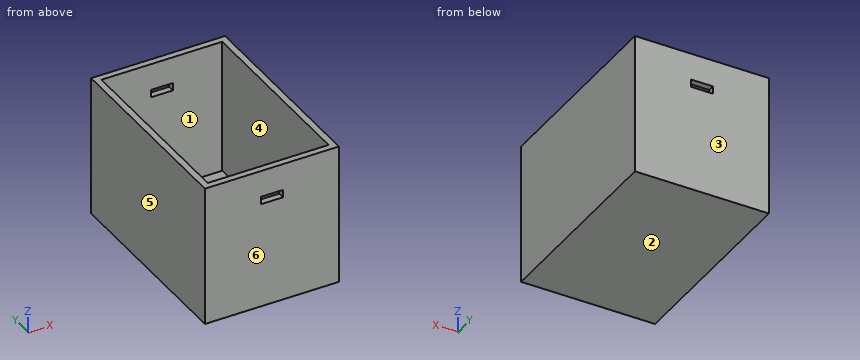
```python
from build123d import *

# Parameters (mm, degrees)
F0_W     = 22
F0_H     = 34
F1_DEPTH = 1.2
F0_W_2   = 24.4
F0_H_2   = 36.4
F2_DEPTH = 25.7
F3_W     = 4
F3_H     = 1.4
F4_DEPTH = 36.401


with BuildPart() as f1:
    # F0 (on Top) → F1 (new body)
    with BuildSketch(Plane.XY):
        Rectangle(F0_W, F0_H)
    extrude(amount=F1_DEPTH)

    # F0 (on Top) → F2 (join)
    with BuildSketch(Plane.XY):
        Rectangle(F0_W_2, F0_H_2)
        Rectangle(F0_W, F0_H, mode=Mode.SUBTRACT)
    extrude(amount=F2_DEPTH)

    # F3 (on face) → F4 (cut, through all)
    with BuildSketch(Plane(origin=(0, 18.2, 0), x_dir=(-1, 0, 0), z_dir=(0, 1, 0))):
        with Locations((0, 20.1)):
            Rectangle(F3_W, F3_H)
    extrude(amount=-F4_DEPTH, mode=Mode.SUBTRACT)


solid = f1.part
```
Part model, mm, in its own coordinate system. Face numbers are marked on the shaded views. A direction names the side the tool comes from. Round coordinates to 2 decimals unless told otherwise and drop trailing zeros. Write each loop counter-clockwise with the first axis right and the second up, starting at its lowest first coordinate (ties: lowest second). Pieces come first, ordered by that corner, then holes. Notation, with made-up numbers: (-6.5, 41) -> (48.5, 41) arc R22 ccw to (48.5, 54) -> close; hole circle Ø5 at (87.5, -4.75). An arc over 180 degrees is marked (long way). Return JSON: item names as keys, results as strings. Group by question number.
Q1. Saw through at D-D on x = 1. Write the cut outline in (y, z).
Q2. Which spindle directions (+Z, -Z, +X, -X, +Y, -Y) get a long thin tool onto all of the face, cutting with end or side? Do the marked faces 1 and 2. Say none if no direction does.
Q3. Mould opens along Y. For the marked faces 3, 4, 5 and 6 say: pulls with the +Y half, pulls with the -Y half, needs draft (parallel to the pull), parting line crosses it, or undercut.
Q4. Saw through at B-B on y = -6. Write the cut outline in (x, z).
Q5. Probe L1, parallel to Y at x = 2.5, z = 18.25; L2, parallel to X at y = -2.5, z = 20.5; L3, parallel to Z at x = -9.75, y = 13. List the from-to ranges inside material, lowest first. Write a range as [from, to].
Q6. Pin check, flat tip, straight feed: pin 1 (2 mm diameter, centred on x = 2, y = 7, fed in from +Z). Stop position of the tip, or through.
Q7. Saw through at A-A on x = 5.25. Write the cut outline in (y, z), plus the area to 3 significant figures.
Q8. Saw through at C-C on z = 6. Write the cut outline in (x, y).
Answer:
{
 "1": {"outline": "(-18.2, 0) -> (18.2, 0) -> (18.2, 19.4) -> (17, 19.4) -> (17, 1.2) -> (-17, 1.2) -> (-17, 19.4) -> (-18.2, 19.4) -> close; (-18.2, 20.8) -> (-17, 20.8) -> (-17, 25.7) -> (-18.2, 25.7) -> close; (17, 20.8) -> (18.2, 20.8) -> (18.2, 25.7) -> (17, 25.7) -> close"},
 "2": {"face 1": "+Z", "face 2": "-Z, +X, -X, +Y, -Y"},
 "3": {"face 3": "pulls with the +Y half", "face 4": "undercut", "face 5": "needs draft", "face 6": "pulls with the -Y half"},
 "4": {"outline": "(-12.2, 0) -> (12.2, 0) -> (12.2, 25.7) -> (11, 25.7) -> (11, 1.2) -> (-11, 1.2) -> (-11, 25.7) -> (-12.2, 25.7) -> close"},
 "5": {"L1": "[-18.2, -17], [17, 18.2]", "L2": "[-12.2, -11], [11, 12.2]", "L3": "[0, 1.2]"},
 "6": {"pin 1": "z = 1.2"},
 "7": {"outline": "(-18.2, 0) -> (18.2, 0) -> (18.2, 25.7) -> (17, 25.7) -> (17, 1.2) -> (-17, 1.2) -> (-17, 25.7) -> (-18.2, 25.7) -> close", "area": "102 mm2"},
 "8": {"outline": "(-12.2, -18.2) -> (12.2, -18.2) -> (12.2, 18.2) -> (-12.2, 18.2) -> close; hole (-11, -17) -> (11, -17) -> (11, 17) -> (-11, 17) -> close"}
}
